Here's the drawing with two shaded views (mm, measured from the low corner). I have some questions. A direction names the side the tool comes from. Give positions to 0.01 mm unless a question says otherwise; leave off trailing zeros. Write each loop counter-clockwise with the first axis right and the second up, starting at its lowest first coordinate (ties: lowest second). Pieces come first, ordered by that corner, then holes. Notation, with made-up numbers: M 33,59 L 89,59 A19 ccw 89,76 Z; hole C -15,0.25 d1. An arc over 180 degrees is marked long. Answer as a JSON object with one key per item and string values. Group by question number.
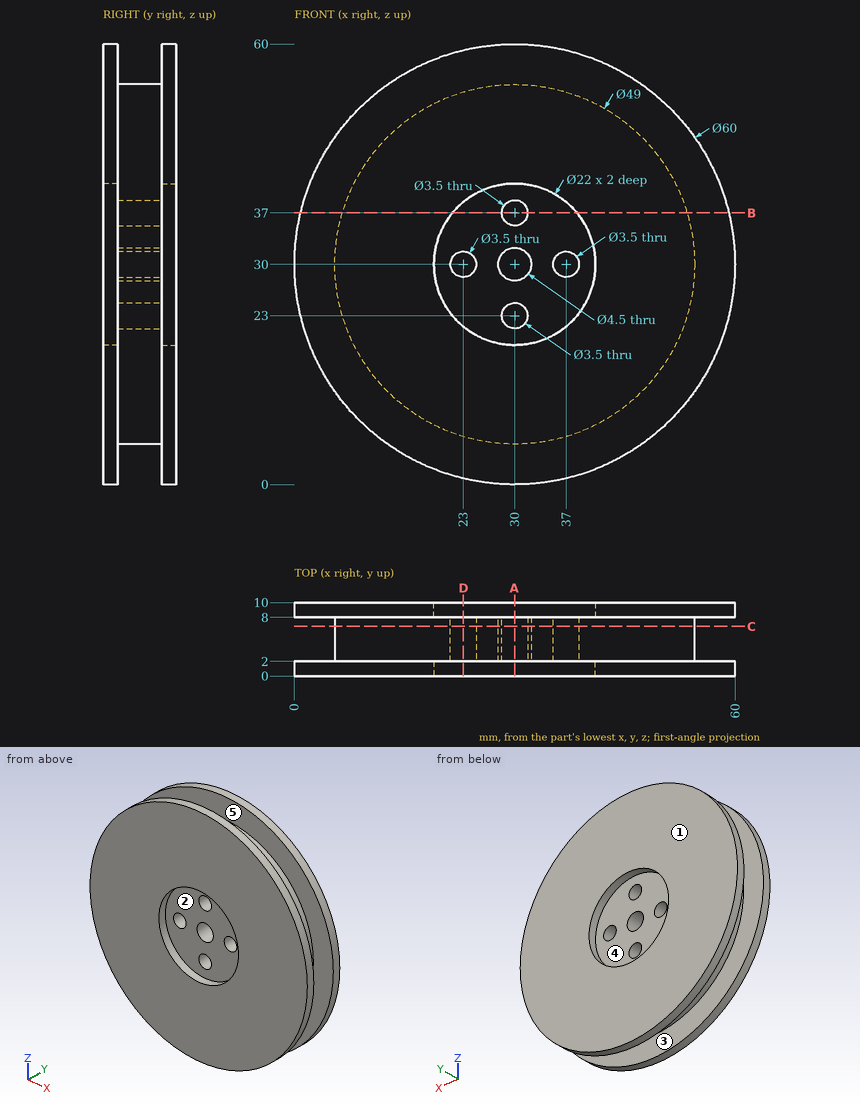
1) I'm going to push flat-ended pins straight in: pin 1 (2 mm diameter, centred on y = 6, z = 25.5, fed in from -X); pin 2 (2.5 mm diameter, centred on x = 30, z = 30, fed in from -Y); pin 3 (6.5 mm diameter, centred on x = 28, z = 26.5, fed in from +Y); pin 4 (1.5 mm diameter, centred on y = 1, z = 25, fed in from +X). Where does each tip first touch, or does it pass through?
2) If we section it at D-D, the plane x = 23: List the corners of the cut face in (y, z) for me.
3) We'd pull the mould along Z, two halves only. Please class the marked faces 4 and 5: released by +Z, released by -Z, zero draft, split by the parting line, or undercut.
4) Please list where these lines run through material, in increasing order: line 1 along Z through (x, y) = (30, 6); line 2 along Y through (x, z) = (17.5, 56); line 3 along Z through (x, y) = (30, 0.85). Write a range as from..to.
5) For the marked faces 1, 2 and 3, which set-ups out of +Z, -Z, +X, -X, +Y, -Y let a thin tool reach every point of the face, with its end or its side?
6) If we section it at C-C, the plane y = 6.75: List the corners of the cut face in (x, z) for me, plus the area to 3 significant figures.
7) If we section it at B-B, the plane z = 37: List the corners of the cut face in (x, y) for me, plus the area to 3 significant figures.
8) If we section it at A-A, the plane x = 30: Give the number of separate pieces and of enclosed holes in the cut face, plus the area to 3 significant figures.
Taken from the geometry:
{
 "1": {"pin 1": "x = 5.75", "pin 2": "through", "pin 3": "y = 8", "pin 4": "x = 59.7"},
 "2": {"outline": "M 0,0.83 L 2,0.83 L 2,6.52 L 8,6.52 L 8,0.83 L 10,0.83 L 10,21.51 L 8,21.51 L 8,28.25 L 2,28.25 L 2,21.51 L 0,21.51 Z; M 0,38.49 L 2,38.49 L 2,31.75 L 8,31.75 L 8,38.49 L 10,38.49 L 10,59.17 L 8,59.17 L 8,53.48 L 2,53.48 L 2,59.17 L 0,59.17 Z"},
 "3": {"face 4": "undercut", "face 5": "zero draft"},
 "4": {"line 1": "5.5..21.25, 24.75..27.75, 32.25..35.25, 38.75..54.5", "line 2": "0..2, 8..10", "line 3": "0..19, 41..60"},
 "5": {"face 1": "+Z, -Z, +X, -X, +Y", "face 2": "-Y", "face 3": "none"},
 "6": {"outline": "C 30,30 d49; hole C 23,30 d3.5; hole C 30,30 d4.5; hole C 30,23 d3.5; hole C 30,37 d3.5; hole C 37,30 d3.5", "area": "1,830 mm²"},
 "7": {"outline": "M 0.83,0 L 21.51,0 L 21.51,2 L 28.25,2 L 28.25,8 L 21.51,8 L 21.51,10 L 0.83,10 L 0.83,8 L 6.52,8 L 6.52,2 L 0.83,2 Z; M 31.75,2 L 38.49,2 L 38.49,0 L 59.17,0 L 59.17,2 L 53.48,2 L 53.48,8 L 59.17,8 L 59.17,10 L 38.49,10 L 38.49,8 L 31.75,8 Z", "area": "426 mm²"},
 "8": {"separate pieces": "4", "enclosed holes": "0", "area": "377 mm²"}
}
